Work out the finished part from the listing and answer in its coordinate system (mm). A direction names the side the tool comes from. Coordinates: 2 decimals unless noted, no trailing zeros. Order: outer loops, then holes, each group sorted by start corner. A loop starts at its lowest first (then second) coordinate and runs counter-clockwise, first axis right, second up. Notation, with made-up numbers: M 84,87 L 116,87 A32 ccw 116,114 Z; hole C -11.5,31.5 d9. An arc over 180 degrees is marked long. Write item = value, one per line. Start each with the question number.
Q1. Find section D-D on x = -220. Give the vertices of the cut face in (y, z), and give its area (3 significant figures).
Q2. A tool of negligible diameter and unlimited length cuts with its end or side. For faces 1 (the flat face through (-86, 11, -3)), 2 (the flat face through (-217.6, 3, -35.1)), 3 (the flat face through (-113, 19, 0)), from which of +Z, -Z, +X, -X, +Y, -Y can it reach the whole face along a straight path? Write none if from no direction.
Q3. Determine the mould class of faces 4 (the cylindrical face through (-220.29, 1.48, -32.77)), 5 (the flat face through (-86, 3, 8)), 6 (the flat face through (-175, 6.2, -0.5)) for opening direction X: released by +X, released by -X, zero draft, split by the parting line, or undercut.
Q4. Straight lines are drawn through the part: line 1 along X through (y, z) = (2.15, 10); line 2 along Z through (x, y) = (-10, 1); line 3 along X through (y, z) = (2, -35). For each, find the intervals that lie inside material, in ascending order.
Q5. Find section C-C on z = 10. Give the vertices of the cut face in (x, y).
Q6. Find section A-A on x = -165. Give the vertices of the cut face in (y, z).
Q7. Find section B-B on z = -35. Give the vertices of the cut face in (x, y).
Q8. Each of these flat-tipped pins is pushed along its axis until it touches: P1, Ø8, axis at y = 5.5, z = 9.5, coming from the -X side; P2, Ø1.5, axis at x = -114, y = 19.5, coming from the -Z side; P3, Ø1.5, axis at x = -131, y = 15.5, coming from the -Z side; P4, Ø3.5, axis at x = -220, z = -35, coming from the -Y side. Where does it stop, or does it pass through?
Autodesk Inventor part; units mm, degrees
ref_plane "作業平面1" through (-115, 0, -25) normal (-1, 0, 0) x (0, 0, 1)
ref_plane "作業平面2" through (-230, 0, 0) normal (0, 0.7071068, 0.7071068) x (-1, 0, 0)
ref_plane "作業平面3" through (-20, 22, 0) normal (0, 1, 0) x (1, 0, 0)
sketch "スケッチ1" plane through (0, 0, 0) normal (0, 1, 0) x (-1, 0, 0)
  line L0 (0, -22) -> (230, -22)
  line L1 (230, -22) -> (230, -25)
  line L2 (230, -25) -> (0, -25)
  line L3 (0, -25) -> (0, -22)
  line L4 (276, 0) -> (-46, 0)
  point P0 (0, 0)
  dimension "d0" = 3
  dimension "d1" = 230
  dimension "d2" = 25
revolve "回転1" add sketch "スケッチ1" angle 90 about axis through (-10, 0, 0) along (1, 0, 0)
sketch "スケッチ2" plane through (-230, 25, 0) normal (0, 0, 1) x (1, 0, 0)
  line L0 (230, 0) -> (0, 0)
  line L1 (0, 0) -> (0, -3)
  line L2 (0, -3) -> (230, -3)
  line L3 (230, -3) -> (230, 0)
  line L4 (230, 0) -> (0, 0)
  line L5 (0, 0) -> (20, 0)
  line L6 (20, 0) -> (20, 20)
  line L7 (20, 20) -> (0, 20)
  line L8 (0, 20) -> (0, 0)
  line L9 (115, 0) -> (115, -3)
  line L10 (0, -3) -> (230, -3)
  line L11 (20, 0) -> (20, -3)
  circle A0 centre (10, 10) radius 2.25
  point P0 (230, -25)
  point P1 (20, 0)
  point P2 (20, -3)
  point P3 (20, 0)
  dimension "d4" = 20
  dimension "d5" = 20
  dimension "d8" = 4.5
extrude "押し出し1" add sketch "スケッチ2" against normal blind 3 contours L11 L2 L1 L0 | L0 L8 L7 L6
ref_plane "作業平面1" through (-115, 0, -25) normal (-1, 0, 0) x (0, 0, 1)
mirror "ミラー1" about plane through (-115, 0, -25) normal (-1, 0, 0) of "押し出し1"
ref_plane "作業平面2" through (-230, 0, 0) normal (0, 0.7071068, 0.7071068) x (-1, 0, 0)
mirror "ミラー2" about plane through (-230, 0, 0) normal (0, 0.7071068, 0.7071068) of "ミラー1", "押し出し1"
ref_plane "作業平面3" through (-20, 22, 0) normal (0, 1, 0) x (1, 0, 0)
sketch "スケッチ4" plane through (-20, 22, 0) normal (0, 1, 0) x (1, 0, 0)
  line L0 (0, 0) -> (20, 0)
  line L1 (20, 0) -> (20, 3)
  line L2 (20, 3) -> (0, 3)
  line L3 (0, 0) -> (0, 3)
  line L4 (20, 0) -> (0, 0)
  line L5 (0, 0) -> (-155, 0)
  line L6 (-155, 0) -> (-155, 3)
  line L7 (-155, 3) -> (0, 3)
  line L8 (0, 3) -> (0, 0)
  line L9 (-210, 0) -> (-210, 22)
  dimension "d22" = 55
extrude "押し出し3" add sketch "スケッチ4" against normal up to surface (22 mm away)
sketch "スケッチ5" plane through (-230, 45, 0) normal (0, 0, 1) x (1, 0, 0)
  line L0 (230, -45) -> (55, -45)
  line L1 (230, -42) -> (210, -42)
  line L2 (230, 0) -> (230, -45)
  line L3 (210, -42) -> (55, -42)
  line L4 (55, -23.2055) -> (55, -45)
  line L5 (55, -23) -> (55, -45)
extrude "押し出し4" add sketch "スケッチ5" along normal blind 17
sketch "スケッチ7" plane through (-175, 3, 0) normal (0, 1, 0) x (1, 0, 0)
  circle A0 centre (165, 35) radius 2.25
  circle A1 centre (165, -10) radius 2.25
  line L0 (0, 0) -> (175, 0)
  line L1 (175, 0) -> (175, -17)
  circle A2 centre (10, -10) radius 2.25
  line L2 (0, 0) -> (0, -17)
  dimension "d23" = 4.5
  dimension "d24" = 10
  dimension "d25" = 10
  dimension "d26" = 4.5
  dimension "d27" = 10
  dimension "d28" = 10
extrude "押し出し6" cut sketch "スケッチ7" against normal up to surface (3 mm away) contours A1 | A2
sketch "スケッチ8" plane through (0, 24.8193, -3) normal (1, 0, 0) x (0, 0, -1)
  arc A0 (19, -24.8193) -> (0, -3.0249) centre (-3, -24.8193) ccw
  line L0 (19, -24.8193) -> (42, -24.8193)
  line L1 (42, -24.8193) -> (42, -21.8193)
  line L2 (21.8193, -21.8193) -> (42, -21.8193)
  arc A1 (21.8193, -21.8193) -> (0, 0) centre (-3, -24.8193) ccw
  line L3 (0, 0) -> (0, 20.1807)
  line L4 (-3, 20.1807) -> (0, 20.1807)
  line L5 (-3, 20.1807) -> (-3, -21.8193)
  line L6 (-3, -21.8193) -> (-20, -21.8193)
  line L7 (-20, -24.8193) -> (-20, -21.8193)
  line L8 (0, -24.8193) -> (-20, -24.8193)
  line L9 (0, -3.0249) -> (0, -24.8193)
  line L10 (-3, 20.1807) -> (-3, -21.8193)
  arc A2 (0, 0) -> (-3, 0.1807) centre (-3, -24.8193) ccw
  point P0 (-3, -24.8193)
  point P1 (-3, 0.1807)
extrude "押し出し7" cut sketch "スケッチ8" against normal up to surface (20 mm away) contours A2 L5 L4 L3
properties part number "CableCoverForFrameHigher"
Findings below:
q1.outline = M 0,-45 L 3,-45 L 3,-37.25 L 0,-37.25 Z; M 0,-32.75 L 3,-32.75 L 3,-24.82 A25 ccw 24.82,-3 L 32.75,-3 L 32.75,0 L 22,0 A22 cw 0,-22 Z; M 37.25,-3 L 45,-3 L 45,0 L 37.25,0 Z
q1.area = 204 mm^2
q2.face_1 = +X, -X, -Y
q2.face_2 = -Z, +X, -X, +Y
q2.face_3 = +Z, +X, -X, +Y
q3.face_4 = undercut
q3.face_5 = zero draft
q3.face_6 = released by -X
q4.line_1 = -175 to -167.25, -162.75 to -12.25, -7.75 to 0
q4.line_2 = -45 to -37.25, -32.75 to -21.98, -3 to 7.75, 12.25 to 17
q4.line_3 = -230 to -222.25, -217.75 to -210, -20 to -12.25, -7.75 to 0
q5.outline = M -175,0 L -167.25,0 L -167.25,3 L -175,3 Z; M -162.75,0 L -12.25,0 L -12.25,3 L -162.75,3 Z; M -7.75,0 L 0,0 L 0,3 L -7.75,3 Z
q6.outline = M 0,-25 A25 ccw 25,0 L 3,0 L 3,7.75 L 0,7.75 L 0,-3 L 21.79,-3 A22 cw 0,-22 Z; M 0,12.25 L 3,12.25 L 3,17 L 0,17 Z
q7.outline = M -230,0 L -222.25,0 L -222.25,3 L -230,3 Z; M -217.75,0 L -210,0 L -210,3 L -217.75,3 Z; M -20,0 L -12.25,0 L -12.25,3 L -20,3 Z; M -7.75,0 L 0,0 L 0,3 L -7.75,3 Z
q8.P1 = -175
q8.P2 = -16.54
q8.P3 = -20.19
q8.P4 = through
